```python
from build123d import *

# Parameters (mm, degrees)
EXTRUDE_1_DEPTH = 20
EXTRUDE_2_DEPTH = 8


with BuildPart() as part:
    # 草图1 → 凸台-拉伸1 (new body)
    with BuildSketch(Plane.XY):
        with BuildLine():
            Line((-6.453218026, -26.118509408), (-6.453218026, -34.118509408))
            ThreePointArc((-6.453218026, -34.118509408), (-5.353218026, -35.218509408), (-4.253218026, -34.118509408))
            Line((-4.253218026, -34.118509408), (-4.253218026, -26.118509408))
            ThreePointArc((-4.253218026, -26.118509408), (-5.353218026, -25.018509408), (-6.453218026, -26.118509408))
        make_face()
    extrude(amount=-EXTRUDE_1_DEPTH)

    # 草图2 → 凸台-拉伸2 (add)
    with BuildSketch(Plane.XY):
        with BuildLine():
            Line((-2.553218026, -34.118509408), (-2.553218026, -26.118509408))
            ThreePointArc((-2.553218026, -26.118509408), (-5.353218026, -23.318509408), (-8.153218026, -26.118509408))
            Line((-8.153218026, -26.118509408), (-8.153218026, -34.118509408))
            ThreePointArc((-8.153218026, -34.118509408), (-5.353218026, -36.918509408), (-2.553218026, -34.118509408))
        make_face()
    extrude(amount=EXTRUDE_2_DEPTH)


solid = part.part
```
The listing builds one solid part. Answer for the finished solid, in the listing's coordinates (mm). A direction names the side the tool comes from. Give positions to 0.01 mm unless a question says otherwise; leave off trailing zeros. Loops run counter-clockwise (first coordinate to the right, second up) from the corner with the lowest first, then second, coordinate; pieces in that order, holes last. Notation, with made-up numbers: (-22, 22) - (3, 22) arc R33 ccw to (3, 60) - close; hole circle Ø2 at (3.5, 75). An arc over 180 degrees is marked (long way). Answer as CSV lines item,"result". Start each with the question number.
Item 1: A cutting plane is placed at A-A on y = -29. Determine the outline of the cut face in (x, z).
Item 2: For faces 1 (the face through (-4.253, -30, -10)), 2 (the face through (-5.33, -25.02, -9.86)), 3 (the face through (-6.453, -30, -10)), 4 (the face through (-5.38, -35.22, -9.86)), 5 (the face through (-8.153, -30, 4)), determine the directions among +Z, -Z, +X, -X, +Y, -Y from which every point of the face is accessible in a straight line to the end or side of a thin tool.
Item 3: Each of these flat-tipped pins is pushed along its axis until it touches: pin 1 (6.5 mm diameter, centred on y = -29.5, z = -11, fed in from +X); pin 2 (6.5 mm diameter, centred on y = -31, z = -12, fed in from -X). Where does it stop, or does it pass through?
Item 4: Find the intervals of material crossed by line 1 (Z direction, x = -6.5, y = -35.75); line 2 (X direction, y = -28, z = -12.25); line 3 (Y direction, x = -5.4, z = -12.25), in increasing order. Write a range as from..to.
Item 5: A cutting plane is placed at B-B on z = 0.5. Determine the outline of the cut face in (x, y).
Item 6: A cutting plane is placed at D-D on z = -3. Determine the outline of the cut face in (x, y).
Item 7: A cutting plane is placed at C-C on x = -5.65. Determine the outline of the cut face in (y, z), then the cut area to 3 significant figures.
Found:
1,outline,"(-8.15, 0) - (-6.45, 0) - (-6.45, -20) - (-4.25, -20) - (-4.25, 0) - (-2.55, 0) - (-2.55, 8) - (-8.15, 8) - close"
2,face 1,"-Z, +X, +Y, -Y"
2,face 2,"-Z, +Y"
2,face 3,"-Z, -X, +Y, -Y"
2,face 4,"-Z, -Y"
2,face 5,"+Z, -Z, -X, +Y, -Y"
3,pin 1,"stops at x = -4.25"
3,pin 2,"stops at x = -6.45"
4,line 1,"z = 0..8"
4,line 2,"x = -6.45..-4.25"
4,line 3,"y = -35.22..-25.02"
5,outline,"(-8.15, -34.12) arc R2.8 ccw to (-2.55, -34.12) - (-2.55, -26.12) arc R2.8 ccw to (-8.15, -26.12) - close"
6,outline,"(-6.45, -34.12) arc R1.1 ccw to (-4.25, -34.12) - (-4.25, -26.12) arc R1.1 ccw to (-6.45, -26.12) - close"
7,outline,"(-36.9, 0) - (-35.18, 0) - (-35.18, -20) - (-25.06, -20) - (-25.06, 0) - (-23.33, 0) - (-23.33, 8) - (-36.9, 8) - close"
7,area,"311 mm^2"
